Here's how the part is built. I have some questions about the finished solid (model axes, mm). A direction names the side the tool comes from. Round coordinates to 2 decimals unless told otherwise and drop trailing zeros. Write each loop counter-clockwise with the first axis right and the second up, starting at its lowest first coordinate (ties: lowest second). Pieces come first, ordered by that corner, then holes. Notation, with made-up numbers: M 37.5,62.5 L 46.5,62.5 A32 ccw 46.5,98.5 Z; hole C 79,15 d3. An arc over 180 degrees is marked long. Use one line per item in the form item = value. Start each with the question number.
Q1. I want a section at A-A on x = 10. List the corners of the cut face in (y, z) for me.
Q2. I need wall thicknesses on line 1 along X through (y, z) = (9, 3.25); line 2 along Z through (x, y) = (10, 26.9); line 3 along X through (y, z) = (17.5, -7.75). Which ranges of each line are inside material? Lowest first, please. Write a range as from..to.
Q3. I want a section at D-D on y = 25.5. List the corners of the cut face in (x, z) for me.
Q4. For faces 1 (the face through (-5, 12, 0)), 2 (the face through (-23, 15, 9)), which set-ups out of +Z, -Z, +X, -X, +Y, -Y let a thin tool reach every point of the face, with its end or its side?
Q5. We'd pull the mould along Z, two halves only. Please class faces 3 (the face through (-8.2, 27.47, -0.08)), 4 (the face through (8, 25, 0)), 5 (the face through (0, 15, -10)): +Z half, -Z half, draft (parallel to the pull), parting line (faces both ways), or undercut.
Q6. I want a section at C-C on z = 0. List the corners of the cut face in (x, y) for me, and give its area (3 significant figures).
Q7. I'm going to push a flat-ended pin straight in: pin 1 Ø1.5 at (x, z) = (-9, -4.5) entering from -Y. Where does the tip first touch, or does it pass through?
Q8. I want a section at B-B on y = 15.75. List the corners of the cut face in (x, z) for me.
```python
from build123d import *

# Parameters (mm, degrees)
SKIZZE1_W                       = 50
SKIZZE1_H                       = 20
AUFSATZ_LINEAR_AUSTRAGEN1_DEPTH = 30
SKIZZE2_W                       = 10
SKIZZE2_H                       = 20
SCHNITT_LINEAR_AUSTRAGEN1_DEPTH = 25
DURCHGANGSLOCH_F_R_M31_D        = 3.6
FASE1_SIZE                      = 3


with BuildPart() as part:
    # Skizze1 → Aufsatz-Linear austragen1 (new body)
    with BuildSketch(Plane(origin=(0, 0, 0), x_dir=(1, 0, 0), z_dir=(0, 1, 0))):
        Rectangle(SKIZZE1_W, SKIZZE1_H)
    extrude(amount=AUFSATZ_LINEAR_AUSTRAGEN1_DEPTH)

    # Skizze2 → Schnitt-Linear austragen1 (cut)
    with BuildSketch(Plane.XZ):
        with Locations((-10, 0)):
            Rectangle(SKIZZE2_W, SKIZZE2_H)
        with Locations((10, 0)):
            Rectangle(SKIZZE2_W, SKIZZE2_H)
    extrude(amount=-SCHNITT_LINEAR_AUSTRAGEN1_DEPTH, mode=Mode.SUBTRACT)

    # Durchgangsloch für M31 (through all)
    with Locations(Plane(origin=(0, 30, 0), x_dir=(1, 0, 0), z_dir=(0, 1, 0))):
        with Locations((-10, 0), (10, 0)):
            Hole(DURCHGANGSLOCH_F_R_M31_D / 2)

    # Fase1
    fase1_edges = [part.edges().sort_by_distance(p)[0] for p in [
        (-25, 15, -10),
        (25, 15, -10),
        (25, 15, 10),
        (-25, 15, 10),
    ]]
    chamfer(fase1_edges, length=FASE1_SIZE)


solid = part.part
```
Reported:
q1.outline = M 25,-10 L 30,-10 L 30,-1.8 L 25,-1.8 Z; M 25,1.8 L 30,1.8 L 30,10 L 25,10 Z
q2.line_1 = -25..-15, -5..5, 15..25
q2.line_2 = -10..-1.8, 1.8..10
q2.line_3 = -24.25..-15, -5..5, 15..24.25
q3.outline = M -25,-7 L -22,-10 L 22,-10 L 25,-7 L 25,7 L 22,10 L -22,10 L -25,7 Z; hole C -10,0 d3.6; hole C 10,0 d3.6
q4.face_1 = +Z, -Z, -Y
q4.face_2 = +Z, -X, +Y, -Y
q5.face_3 = undercut
q5.face_4 = draft
q5.face_5 = -Z half
q6.outline = M -25,0 L -15,0 L -15,25 L -11.8,25 L -11.8,30 L -25,30 Z; M -8.2,25 L -5,25 L -5,0 L 5,0 L 5,25 L 8.2,25 L 8.2,30 L -8.2,30 Z; M 11.8,25 L 15,25 L 15,0 L 25,0 L 25,30 L 11.8,30 Z
q6.area = 964 mm^2
q7.pin_1 = 25
q8.outline = M -25,-7 L -22,-10 L -15,-10 L -15,10 L -22,10 L -25,7 Z; M -5,-10 L 5,-10 L 5,10 L -5,10 Z; M 15,-10 L 22,-10 L 25,-7 L 25,7 L 22,10 L 15,10 Z
